from build123d import *

# Parameters (mm, degrees)
SKETCH1_W                                      = 100
SKETCH1_H                                      = 150
BOSS_EXTRUDE1_DEPTH                            = 2.5
CSK_FOR_M5_FLAT_HEAD_MACHINE_SCREW1_AT_2_COUNT = 2
CSK_FOR_M5_FLAT_HEAD_MACHINE_SCREW1_AT_2_PITCH = 85
CSK_FOR_M5_FLAT_HEAD_MACHINE_SCREW1_AT_3_COUNT = 2
CSK_FOR_M5_FLAT_HEAD_MACHINE_SCREW1_AT_3_PITCH = 159.530561335
CSK_FOR_M5_FLAT_HEAD_MACHINE_SCREW1_AT_4_COUNT = 2
CSK_FOR_M5_FLAT_HEAD_MACHINE_SCREW1_AT_4_PITCH = 135
SKETCH5_W                                      = 110
SKETCH5_H                                      = 160
SKETCH5_W_2                                    = 100
SKETCH5_H_2                                    = 150
BOSS_EXTRUDE2_DEPTH                            = 10
SKETCH6_W                                      = 12.7
SKETCH6_H                                      = 5
CUT_EXTRUDE1_DEPTH                             = 5
FILLET1_R                                      = 6
CUT_EXTRUDE2_DEPTH                             = 98.59610648
CUT_EXTRUDE2_DEPTH_BACK                        = 98.59610648
SKETCH7_R                                      = 37.5
CHAMFER2_SIZE                                  = 1


with BuildPart() as part:
    # Sketch1 → Boss-Extrude1 (new, symmetric)
    with BuildSketch(Plane(origin=(0, 0, 0), x_dir=(1, 0, 0), z_dir=(0, 1, 0))):
        Rectangle(SKETCH1_W, SKETCH1_H)
    extrude(amount=BOSS_EXTRUDE1_DEPTH, both=True)

    # Sketch4 → CSK for M5 Flat Head Machine Screw1 (revolve, cut)
    with BuildSketch(Plane(origin=(-42.5, 2.5, -67.5), x_dir=(0, 0, 1), z_dir=(1, 0, 0))):
        Polygon((0, 0), (0, 5), (2.75, 5), (2.75, 2.45), (5.2, 0), align=None)
    csk_for_m5_flat_head_machine_screw1 = revolve(axis=Axis((-42.5, 8.85, -67.5), (0, -1, 0)), mode=Mode.SUBTRACT)

    # CSK for M5 Flat Head Machine Screw1 at 2: CSK for M5 Flat Head Machine Screw1 ×2
    with Locations(*[(i * CSK_FOR_M5_FLAT_HEAD_MACHINE_SCREW1_AT_2_PITCH, 0, 0) for i in range(1, CSK_FOR_M5_FLAT_HEAD_MACHINE_SCREW1_AT_2_COUNT)]):
        add(csk_for_m5_flat_head_machine_screw1, mode=Mode.SUBTRACT)

    # CSK for M5 Flat Head Machine Screw1 at 3: CSK for M5 Flat Head Machine Screw1 ×2
    with Locations(*[Vector(0.5328132696861391, 0, 0.8462328400897507) * (i * CSK_FOR_M5_FLAT_HEAD_MACHINE_SCREW1_AT_3_PITCH) for i in range(1, CSK_FOR_M5_FLAT_HEAD_MACHINE_SCREW1_AT_3_COUNT)]):
        add(csk_for_m5_flat_head_machine_screw1, mode=Mode.SUBTRACT)

    # CSK for M5 Flat Head Machine Screw1 at 4: CSK for M5 Flat Head Machine Screw1 ×2
    with Locations(*[(0, 0, i * CSK_FOR_M5_FLAT_HEAD_MACHINE_SCREW1_AT_4_PITCH) for i in range(1, CSK_FOR_M5_FLAT_HEAD_MACHINE_SCREW1_AT_4_COUNT)]):
        add(csk_for_m5_flat_head_machine_screw1, mode=Mode.SUBTRACT)

    # Sketch5 → Boss-Extrude2 (add)
    with BuildSketch(Plane(origin=(0, 2.5, 0), x_dir=(1, 0, 0), z_dir=(0, 1, 0))):
        Rectangle(SKETCH5_W, SKETCH5_H)
        Rectangle(SKETCH5_W_2, SKETCH5_H_2, mode=Mode.SUBTRACT)
    extrude(amount=-BOSS_EXTRUDE2_DEPTH)

    # Sketch6 → Cut-Extrude1 (cut)
    with BuildSketch(Plane.XZ.offset(7.5)):
        with Locations((0, 77.5)):
            Rectangle(SKETCH6_W, SKETCH6_H)
    extrude(amount=-CUT_EXTRUDE1_DEPTH, mode=Mode.SUBTRACT)

    # Fillet1
    fillet1_edges = [part.edges().sort_by_distance(p)[0] for p in [
        (55, -2.5, -80),
        (55, -2.5, 80),
        (-55, -2.5, 80),
        (-55, -2.5, -80),
        (-50, -5, -75),
        (50, -5, -75),
        (50, -5, 75),
        (-50, -5, 75),
    ]]
    fillet(fillet1_edges, radius=FILLET1_R)

    # Sketch7 → Cut-Extrude2 (cut, two sides: drawn at the far end of the back side and taken through both)
    with BuildSketch(Plane(origin=(0, 2.5, 0), x_dir=(1, 0, 0), z_dir=(0, 1, 0)).offset(-CUT_EXTRUDE2_DEPTH_BACK)):
        with Locations(Location((0, 0, 0), (0, 0, 90))):
            Circle(SKETCH7_R)
    extrude(amount=CUT_EXTRUDE2_DEPTH + CUT_EXTRUDE2_DEPTH_BACK, mode=Mode.SUBTRACT)

    # Chamfer2
    chamfer2_edges = [part.edges().sort_by_distance(p)[0] for p in [
        (-48.242640687, -7.5, -73.242640687),
        (48.242640687, -7.5, -73.242640687),
        (48.242640687, -7.5, 73.242640687),
        (-48.242640687, -7.5, 73.242640687),
        (0, 2.5, 37.5),
        (0, -2.5, 37.5),
        (25.175, -7.5, 75),
        (6.35, -7.5, 77.5),
        (-6.35, -7.5, 77.5),
        (0, 2.5, 80),
        (55, 2.5, 0),
        (0, 2.5, -80),
        (-55, 2.5, 0),
        (-53.242640687, 2.5, 78.242640687),
        (-53.242640687, 2.5, -78.242640687),
        (53.242640687, 2.5, -78.242640687),
        (53.242640687, 2.5, 78.242640687),
        (50, -7.5, 0),
        (0, -7.5, -75),
        (-50, -7.5, 0),
        (-25.175, -7.5, 75),
    ]]
    chamfer(chamfer2_edges, length=CHAMFER2_SIZE)


solid = part.part
The model under review builds one solid part; all positions refer to its coordinate system, in mm. A direction names the side the tool comes from. Give positions to 0.01 mm unless a question says otherwise; leave off trailing zeros. Order: outer loops, then holes, each group sorted by start corner. A loop starts at its lowest first (then second) coordinate and runs counter-clockwise, first axis right, second up. Notation, with made-up numbers: M 35,56 L 70,56 A18 cw 70,78 Z; hole C 30.5,85 d9. An arc over 180 degrees is marked long. Use one line per item in the form item = value. Start each with the question number.
Item 1: The part is to be moulded in two halves that separate along X. For faces 1 (the flat face through (-1, -4, -75)), 2 (the flat face through (-37, 2.5, -19)), 3 (the conical face through (-52.696, 2.215, -77.778)), say which applies: pulls with the +X half, pulls with the -X half, needs draft (parallel to the pull), parting line crosses it, or undercut.
Item 2: We need section B-B on x = 0. Give the boundary of the cut face in (y, z).
Item 3: For faces 4 (the flat face through (-6.35, -5, 77)), 5 (the cylindrical face through (48.196, -4.528, 73.289)), 6 (the conical face through (-52.778, 2.215, 77.696)), list the 3-axis set-ups (+Z, -Z, +X, -X, +Y, -Y) from which the entire face can be reached by the end or side of a thin tool; tool diameter is ignored.
Item 4: We need section A-A on z = 0. Give the boundary of the cut face in (x, y).
Item 5: To check wall thickness, follow line 1 along X through (y, z) = (-1.15, -67.5); line 2 along Z through (x, y) = (-42.5, -0.8); line 3 along X through (y, z) = (0.6, 0). State the ranges of each line that lie inside material, in increasing order. Write a range as from..to.
Item 6: Insertion check: pin 1 Ø9 at (x, z) = (-42.5, -67.5) entering from +Y; pin 2 Ø4.5 at (y, z) = (-4.5, 78) entering from -X; pin 3 Ø6.5 at (x, z) = (42.5, -67.5) entering from -Y. Each pin has a flat end and moves straight along its axis. Give the tip position at first contact, or say it passes through.
Item 7: We need section C-C on y = -4.75. Give the boundary of the cut face in (x, z).
Completed:
q1.face_1 = undercut
q1.face_2 = needs draft
q1.face_3 = pulls with the -X half
q2.outline = M -7.5,-80 L 1.5,-80 L 2.5,-79 L 2.5,-38.5 L 1.5,-37.5 L -1.5,-37.5 L -2.5,-38.5 L -2.5,-75 L -6.5,-75 L -7.5,-76 Z; M -2.5,38.5 L -1.5,37.5 L 1.5,37.5 L 2.5,38.5 L 2.5,79 L 1.5,80 L -2.5,80 Z
q3.face_4 = +Z, -Y
q3.face_5 = -Y
q3.face_6 = +Z, -X, +Y
q4.outline = M -55,-7.5 L -51,-7.5 L -50,-6.5 L -50,-2.5 L -38.5,-2.5 L -37.5,-1.5 L -37.5,1.5 L -38.5,2.5 L -54,2.5 L -55,1.5 Z; M 37.5,-1.5 L 38.5,-2.5 L 50,-2.5 L 50,-6.5 L 51,-7.5 L 55,-7.5 L 55,1.5 L 54,2.5 L 38.5,2.5 L 37.5,1.5 Z
q5.line_1 = -55..-45.25, -39.75..39.75, 45.25..55
q5.line_2 = -80..-70.25, -64.75..64.75, 70.25..80
q5.line_3 = -55..-37.5, 37.5..55
q6.pin_1 = 1.8
q6.pin_2 = -54.74
q6.pin_3 = -2.5
q7.outline = M -55,-74 A6 ccw -49,-80 L 49,-80 A6 ccw 55,-74 L 55,74 A6 ccw 49,80 L 6.35,80 L 6.35,75 L 44,75 A6 cw 50,69 L 50,-69 A6 cw 44,-75 L -44,-75 A6 cw -50,-69 L -50,69 A6 cw -44,75 L -6.35,75 L -6.35,80 L -49,80 A6 ccw -55,74 Z
